```python
from build123d import *

# Parameters (mm, degrees)
SKETCH1_R           = 3
BOSS_EXTRUDE1_DEPTH = 200
REVOLVE1_ANGLE      = 180
REVOLVE2_ANGLE      = 180


with BuildPart() as part:
    # Sketch1 → Boss-Extrude1 (new body)
    with BuildSketch(Plane.XY):
        Circle(SKETCH1_R)
    extrude(amount=BOSS_EXTRUDE1_DEPTH)

    # Sketch2 → Revolve1 (revolve)
    with BuildSketch(Plane.XY.offset(200)):
        with BuildLine():
            Line((0, 8), (0, 7))
            Line((0, 7), (0, -7))
            Line((0, -7), (0, -8))
            ThreePointArc((0, -8), (8, 0), (0, 8))
        make_face()
    revolve(axis=Axis((0, 8, 200), (0, 1, 0)), revolution_arc=REVOLVE1_ANGLE)

    # Sketch3 → Cut-Revolve1 (revolve, cut)
    with BuildSketch(Plane.XY.offset(200)):
        with BuildLine():
            Line((0, 7), (0, -7))
            ThreePointArc((0, -7), (7, 0), (0, 7))
        make_face()
    revolve(axis=Axis((0, 7, 200), (0, -1, 0)), mode=Mode.SUBTRACT)

    # Sketch4 → Revolve2 (revolve)
    with BuildSketch(Plane(origin=(0, 0, 0), x_dir=(-1, 0, 0), z_dir=(0, 0, -1))):
        with BuildLine():
            Line((0, 8), (0, -8))
            ThreePointArc((0, -8), (8, 0), (0, 8))
        make_face()
    revolve(axis=Axis((0, 8, 0), (0, 1, 0)), revolution_arc=REVOLVE2_ANGLE)

    # Sketch5 → Cut-Revolve2 (revolve, cut)
    with BuildSketch(Plane(origin=(0, 0, 0), x_dir=(-1, 0, 0), z_dir=(0, 0, -1))):
        with BuildLine():
            Line((0, 7), (0, -7))
            ThreePointArc((0, -7), (7, 0), (0, 7))
        make_face()
    revolve(axis=Axis((0, 7, 0), (0, -1, 0)), mode=Mode.SUBTRACT)


solid = part.part
```
For this review, take the finished solid that the model builds, in its own axes (mm). Coordinates: 2 decimals unless noted, no trailing zeros. Write each loop counter-clockwise with the first axis right and the second up, starting at its lowest first coordinate (ties: lowest second). Pieces come first, ordered by that corner, then holes. Notation, with made-up numbers: (-1.75, 19) - (46.25, 19) arc R24 ccw to (46.25, 46) - close; hole circle Ø11 at (55.25, 88). An arc over 180 degrees is marked (long way). Put each result on its own line as item: value.
1. Add section C-C, the plane z = 112.5. Give the boundary of the cut face in (x, y), then the cut area to 3 significant figures.
Values found:
outline: circle Ø6 at (0, 0)
area: 28.3 mm²
2. For pin 1 (5 mm diameter, centred on x = 2, z = 38, fed in from -Y); pin 2 (1 mm diameter, centred on y = 2.5, z = 108.5, fed in from +X); pin 3 (1 mm diameter, centred on x = 3, y = -5, fed in from -Z), all flat-tipped, find the tip position at first contact; note any pin that passes through.
Values found:
pin 1: y = -3
pin 2: x = 2.24
pin 3: z = 2.99
3. Mouldability with a two-part tool opening along Z and no side actions: class faces 1 (the flat face through (-4, -6, 0)), 2 (the cylindrical face through (-3, 0, 99)), 3 (the flat face through (4, -6, 200)) as released by +Z, released by -Z, zero draft, split by the parting line, or undercut.
Values found:
face 1: released by -Z
face 2: undercut
face 3: released by +Z
4. Add section A-A, the plane y = 0. Give the boundary of the cut face in (x, z), then the cut area to 3 significant figures.
Values found:
outline: (-8, 0) - (-7, 0) arc R7 cw to (7, 0) - (8, 0) arc R8 ccw to (3, 7.42) - (3, 192.58) arc R8 ccw to (8, 200) - (7, 200) arc R7 cw to (-7, 200) - (-8, 200) arc R8 ccw to (-3, 192.58) - (-3, 7.42) arc R8 ccw to start
area: 1,150 mm²
5. Add section B-B, the plane x = 4.75. Give the boundary of the cut face in (y, z).
Values found:
outline: (-6.44, 0) - (-5.14, 0) arc R5.14 cw to (5.14, 0) - (6.44, 0) arc R6.44 ccw to start; (-6.44, 200) arc R6.44 ccw to (6.44, 200) - (5.14, 200) arc R5.14 cw to (-5.14, 200) - close
6. Wall thickness on probe 1 along Z at (x, y) = (-4, -2.5); probe 2 along Z at (x, y) = (5, 0) (3 decimals); probe 3 along Y at (x, z) = (-0.25, 131): over which ranges is each line inside the solid? List them lowest first.
Values found:
probe 1: 5.17 to 6.46, 193.54 to 194.83
probe 2: 4.899 to 6.245, 193.755 to 195.101
probe 3: -2.99 to 2.99
